CAD build for the part. Positions are in the model's coordinates, mm. Face numbers are marked on the shaded views. Coordinates: 2 decimals unless noted, no trailing zeros. Order: outer loops, then holes, each group sorted by start corner. A loop starts at its lowest first (then second) coordinate and runs counter-clockwise, first axis right, second up. Notation, with made-up numbers: M 84.25,-35 L 92.25,-35 A21 ccw 92.25,-31 Z; hole C -9.75,86.5 d4. An arc over 180 degrees is marked long. One line per item, written item: value.
Autodesk Inventor part; units mm, degrees
ref_plane "YZ Plane" through (0, 0, 0) normal (1, 0, 0) x (0, 1, 0)
ref_plane "XZ Plane" through (0, 0, 0) normal (0, 1, 0) x (-1, 0, 0)
ref_plane "Work Plane1" through (0, 0, 18) normal (0, 0, 1) x (1, 0, 0)
sketch "Sketch1" plane through (0, 0, 0) normal (1, 0, 0) x (0, 1, 0)
  arc A0 (-3.5373, 37.5621) -> (-14.976, 34) centre (-8.702, 34) ccw
  line L0 (0, 54.2276) -> (0, -32.966) construction
  line L1 (0, -32.966) -> (0, 54.2276)
  line L2 (-24.1835, 0) -> (27.9587, 0) construction
  line L3 (-14.976, 0) -> (-14.976, 34)
  line L4 (-24.1835, 18) -> (27.9587, 18) construction
  arc A1 (-2.428, 34) -> (-14.976, 34) centre (-8.702, 34) ccw
  arc A2 (-2.335, 24) -> (0.4081, 18.7817) centre (4, 24) ccw
  line L5 (-0.319, 19.362) -> (-0.4473, 19.4885)
  line L6 (-2.335, 24) -> (-2.428, 34)
  line L7 (9.2809, 11.7535) -> (0.4081, 18.7817)
  arc A3 (-14.976, 0) -> (9.2809, 11.7535) centre (0, 0) ccw
  line L8 (9.5142, 12.0484) -> (0.6316, 19.0844)
  arc A4 (-1.959, 24.0017) -> (0.6316, 19.0844) centre (4, 24) ccw
  line L9 (-1.959, 24.0017) -> (-2.052, 34.0018)
  arc A5 (-2.052, 34.0018) -> (-15.352, 34) centre (-8.702, 34) ccw
  line L10 (-15.352, 34) -> (-15.352, 0)
  arc A6 (-15.352, 0) -> (9.5142, 12.0484) centre (0, 0) ccw
  dimension "d2" = 12.548
  dimension "d3" = 34
  dimension "d4" = 8.702
  dimension "d8" = 12.67
  dimension "d9" = 4
  dimension "d10" = 6
  dimension "d11" = 29.952
  dimension "d12" = 0.376
extrude "Extrusion1" add sketch "Sketch1" along normal mid plane 6 contours A0 L3 A3 L1 A6 L10 A5 L9 A4 A2 L6 A1 | A3 L7 A2 L1 A4 L8 A6
equation "\"start\" = d3"
equation "\"d7\" = start"
properties part number "paseknowy"
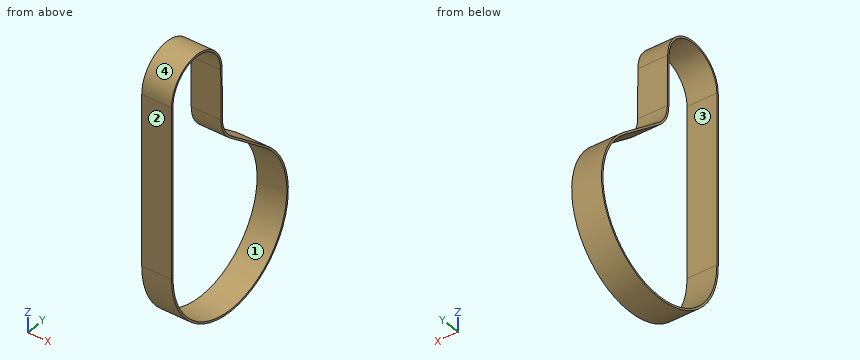
Q1. Pin check, flat tips, straight feed: pin 1 Ø1 at (x, z) = (-1.5, 23.5) entering from +Y; pin 2 Ø1.8 at (x, z) = (-1, 23) entering from +Y; pin 3 Ø2 at (x, y) = (0, 9.5) entering from +Z. Stop position of each tip, or through.
Recorded:
pin 1: stops at y = -1.87
pin 2: stops at y = -1.65
pin 3: stops at z = 12.85
Q2. Slice it at A-A (z = 11). List the corners of the cut face in (x, y).
Recorded:
outline: M -3,-15.35 L 3,-15.35 L 3,-14.98 L -3,-14.98 Z; M -3,10.16 L 3,10.16 L 3,10.71 L -3,10.71 Z
Q3. Slice it at B-B (y = 6). List the corners of the cut face in (x, z).
Recorded:
outline: M -3,-14.13 L 3,-14.13 L 3,-13.72 L -3,-13.72 Z; M -3,14.35 L 3,14.35 L 3,14.83 L -3,14.83 Z
Q4. Mould opens along Z. For the marked faces 1, 2, 3 and 4 say: released by +Z, released by -Z, zero draft, split by the parting line, or undercut.
Recorded:
face 1: undercut
face 2: zero draft
face 3: undercut
face 4: released by +Z
Q5. Drill centre lines: line 1 along Y through (x, z) = (-1.2, 24) (3 decimals); line 2 along Y through (x, z) = (-2.7, 33); line 3 along Z through (x, y) = (-0.6, -5). Where is each one in solid material? Low to high.
Recorded:
line 1: y = -15.352 to -14.976, -2.335 to -1.959
line 2: y = -15.35 to -14.98, -2.42 to -2.04
line 3: z = -14.51 to -14.12, 39.07 to 39.52
